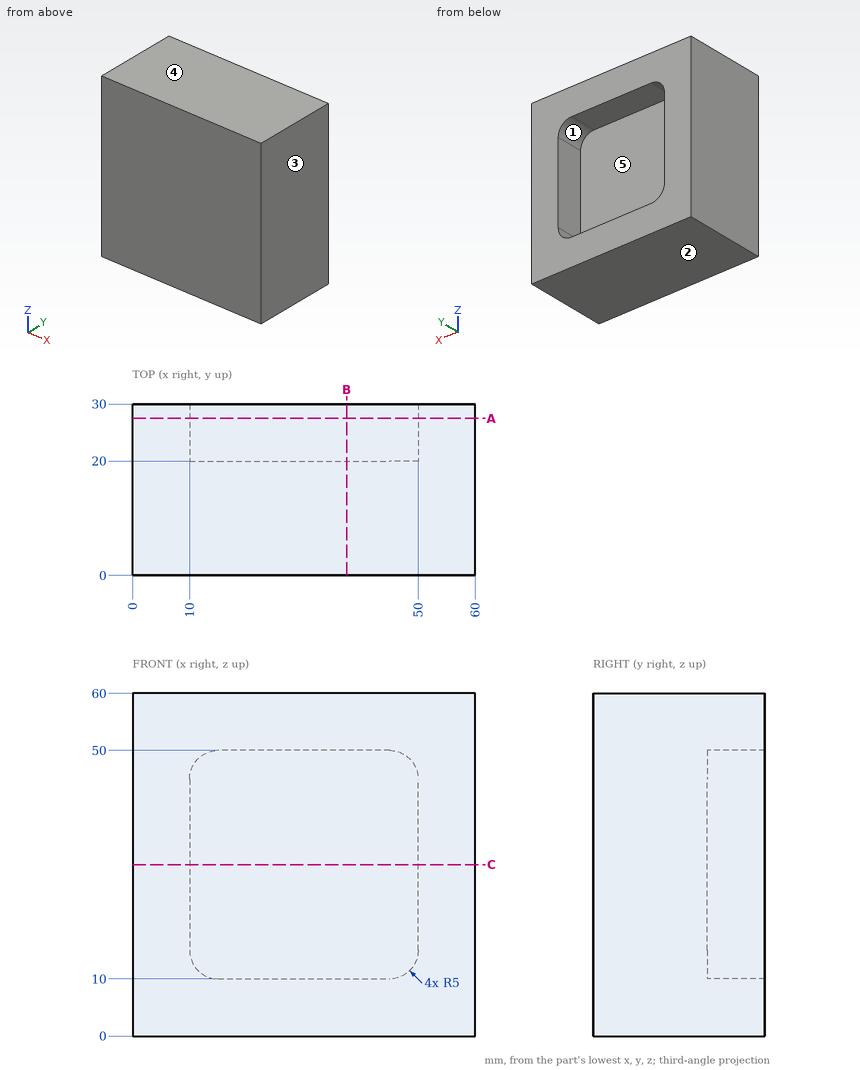
Part print with two shaded views. Sizes in mm from the minimum x, y, z corner. A direction names the side the tool comes from. Round coordinates to 2 decimals unless told otherwise and drop trailing zeros. Loops run counter-clockwise (first coordinate to the right, second up) from the corner with the lowest first, then second, coordinate; pieces in that order, holes last. Notation, with made-up numbers: M 70,-24 L 113,-24 A10 ccw 113,-15 Z; hole C 51,80 d6. An arc over 180 degrees is marked long. Return JSON: item names as keys, results as strings. Group by question number.
(1) Tool access for the marked faces 4 and 5: list every direction of +Z, -Z, +X, -X, +Y, -Y with a clear straight run to the whole face (end or side of a thin tool).
(2) Saw through at B-B, the plane x = 37.5. List the corners of the cut face in (y, z).
(3) Wall check: probe 1 along Z at (x, y) = (29, 27.5); probe 2 along Y at (x, z) = (44, 12). Give the ranges that are in metal, low to high. Write a range as [from, to].
(4) Mould opens along Z. For the marked faces 1, 2 and 3 say: +Z half, -Z half, draft (parallel to the pull), parting line (faces both ways), or undercut.
(5) Saw through at A-A, the plane y = 27.5. List the corners of the cut face in (x, z), and give its area (3 significant figures).
(6) Drop a flat-ended pin along its axis: P1, Ø20, axis at x = 31, z = 35.5, coming from the +Y side. Give the stop position or say it passes through.
(7) Saw through at C-C, the plane z = 30. List the corners of the cut face in (x, y).
Answer list:
{
 "1": {"face 4": "+Z, +X, -X, +Y, -Y", "face 5": "+Y"},
 "2": {"outline": "M 0,0 L 30,0 L 30,10 L 20,10 L 20,50 L 30,50 L 30,60 L 0,60 Z"},
 "3": {"probe 1": "[0, 10], [50, 60]", "probe 2": "[0, 20]"},
 "4": {"face 1": "undercut", "face 2": "-Z half", "face 3": "draft"},
 "5": {"outline": "M 0,0 L 60,0 L 60,60 L 0,60 Z; hole M 10,15 A5 ccw 15,10 L 45,10 A5 ccw 50,15 L 50,45 A5 ccw 45,50 L 15,50 A5 ccw 10,45 Z", "area": "2,020 mm2"},
 "6": {"P1": "y = 20"},
 "7": {"outline": "M 0,0 L 60,0 L 60,30 L 50,30 L 50,20 L 10,20 L 10,30 L 0,30 Z"}
}
